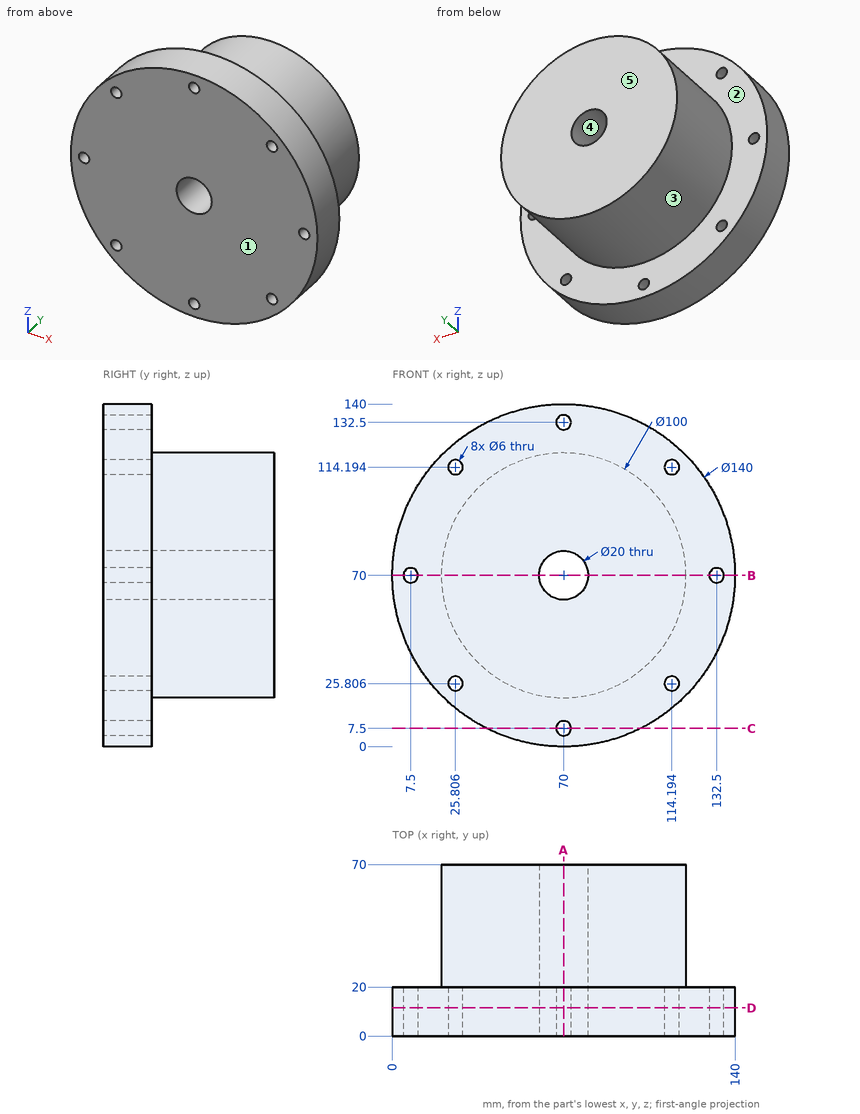
The figure shows three views and two pictorial views of one solid part (mm, origin at its lowest corner). Answer the questions. A direction names the side the tool comes from. Round coordinates to 2 decimals unless told otherwise and drop trailing zeros. Order: outer loops, then holes, each group sorted by start corner. A loop starts at its lowest first (then second) coordinate and runs counter-clockwise, first axis right, second up.
Q1. A cutting plane is placed at C-C, the plane z = 7.5. Determine the outline of the cut face in (x, y).
Solution:
outline: (38.48, 0) - (67, 0) - (67, 20) - (38.48, 20) - close; (73, 0) - (101.52, 0) - (101.52, 20) - (73, 20) - close
Q2. A cutting plane is placed at A-A, the plane x = 70. Determine the outline of the cut face in (y, z).
Solution:
outline: (0, 0) - (20, 0) - (20, 4.5) - (0, 4.5) - close; (0, 10.5) - (20, 10.5) - (20, 20) - (70, 20) - (70, 60) - (0, 60) - close; (0, 80) - (70, 80) - (70, 120) - (20, 120) - (20, 129.5) - (0, 129.5) - close; (0, 135.5) - (20, 135.5) - (20, 140) - (0, 140) - close
Q3. A cutting plane is placed at B-B, the plane z = 70. Determine the outline of the cut face in (x, y).
Solution:
outline: (0, 0) - (4.5, 0) - (4.5, 20) - (0, 20) - close; (10.5, 0) - (60, 0) - (60, 70) - (20, 70) - (20, 20) - (10.5, 20) - close; (80, 0) - (129.5, 0) - (129.5, 20) - (120, 20) - (120, 70) - (80, 70) - close; (135.5, 0) - (140, 0) - (140, 20) - (135.5, 20) - close
Q4. Given pin 1 Ø8 at (x, y) = (58, 49.5) entering from +Z; pin 2 Ø1 at (x, z) = (32.5, 112) entering from +Y; pin 3 Ø2 at (y, z) = (22.5, 28.5) entering from +X, each flat-ended and moving along its own axis, determine where each tip first touches the part or whether it passes through.
Solution:
pin 1: stops at z = 119.36
pin 2: stops at y = 20
pin 3: stops at x = 99.32
Q5. A cutting plane is placed at D-D, the plane y = 11.5. Count the separate pieces of the cut face and the enclosed holes in it, then the cut area to 3 significant figures.
Solution:
separate pieces: 1
enclosed holes: 9
area: 14,900 mm2
Q6. Find the intervals of material crossed by line 1 along Y through (x, z) = (64.5, 19); line 2 along Z through (x, y) = (73, 58); line 3 along Z through (x, y) = (82.5, 34.5), in increasing order.
Solution:
line 1: y = 0 to 20
line 2: z = 20.09 to 60.46, 79.54 to 119.91
line 3: z = 21.59 to 118.41
Q7. The mould has two halves that part along X. Classify the marked faces 3, 4 and 5: pulls with the +X half, pulls with the -X half, needs draft (parallel to the pull), parting line crosses it, or undercut.
Solution:
face 3: parting line crosses it
face 4: undercut
face 5: needs draft
Q8. A tool of negligible diameter and unlimited length cuts with its end or side. For the marked faces 1 and 2, from which of +Z, -Z, +X, -X, +Y, -Y can it reach the whole face along a straight path? Write none if from no direction.
Solution:
face 1: +Z, -Z, +X, -X, -Y
face 2: +Y
